from build123d import *

# Parameters (mm, degrees)
SKETCH_1_W          = 9
SKETCH_1_H          = 6.5
EXTRUDE_1_DEPTH     = 400
SKETCH_2_R          = 1.75
CUT_EXTRUDE_1_DEPTH = 7.5
SKETCH_3_R          = 3
CUT_EXTRUDE_2_DEPTH = 3.5
CUT_EXTRUDE_3_DEPTH = 401
SKETCH_5_R          = 1.75
CUT_EXTRUDE_4_DEPTH = 10


with BuildPart() as part:
    # 草图1 → 凸台-拉伸1 (new body)
    with BuildSketch(Plane.XY):
        Rectangle(SKETCH_1_W, SKETCH_1_H)
    extrude(amount=EXTRUDE_1_DEPTH)

    # 草图2 → 切除-拉伸1 (cut, through all)
    with BuildSketch(Plane(origin=(0, 3.25, 0), x_dir=(1, 0, 0), z_dir=(0, 1, 0))):
        with Locations((0, -7.5)):
            Circle(SKETCH_2_R)
        with Locations((0, -27.5)):
            Circle(SKETCH_2_R)
        with Locations((0, -47.5)):
            Circle(SKETCH_2_R)
        with Locations((0, -67.5)):
            Circle(SKETCH_2_R)
        with Locations((0, -87.5)):
            Circle(SKETCH_2_R)
        with Locations((0, -107.5)):
            Circle(SKETCH_2_R)
        with Locations((0, -127.5)):
            Circle(SKETCH_2_R)
        with Locations((0, -147.5)):
            Circle(SKETCH_2_R)
        with Locations((0, -167.5)):
            Circle(SKETCH_2_R)
        with Locations((0, -187.5)):
            Circle(SKETCH_2_R)
        with Locations((0, -207.5)):
            Circle(SKETCH_2_R)
        with Locations((0, -227.5)):
            Circle(SKETCH_2_R)
        with Locations((0, -247.5)):
            Circle(SKETCH_2_R)
        with Locations((0, -267.5)):
            Circle(SKETCH_2_R)
        with Locations((0, -287.5)):
            Circle(SKETCH_2_R)
        with Locations((0, -307.5)):
            Circle(SKETCH_2_R)
        with Locations((0, -327.5)):
            Circle(SKETCH_2_R)
        with Locations((0, -347.5)):
            Circle(SKETCH_2_R)
        with Locations((0, -367.5)):
            Circle(SKETCH_2_R)
    extrude(amount=-CUT_EXTRUDE_1_DEPTH, mode=Mode.SUBTRACT)

    # 草图3 → 切除-拉伸2 (cut)
    with BuildSketch(Plane(origin=(0, 3.25, 0), x_dir=(1, 0, 0), z_dir=(0, 1, 0))):
        with Locations((0, -7.5)):
            Circle(SKETCH_3_R)
        with Locations((0, -27.5)):
            Circle(SKETCH_3_R)
        with Locations((0, -47.5)):
            Circle(SKETCH_3_R)
        with Locations((0, -67.5)):
            Circle(SKETCH_3_R)
        with Locations((0, -87.5)):
            Circle(SKETCH_3_R)
        with Locations((0, -107.5)):
            Circle(SKETCH_3_R)
        with Locations((0, -127.5)):
            Circle(SKETCH_3_R)
        with Locations((0, -147.5)):
            Circle(SKETCH_3_R)
        with Locations((0, -167.5)):
            Circle(SKETCH_3_R)
        with Locations((0, -187.5)):
            Circle(SKETCH_3_R)
        with Locations((0, -207.5)):
            Circle(SKETCH_3_R)
        with Locations((0, -227.5)):
            Circle(SKETCH_3_R)
        with Locations((0, -247.5)):
            Circle(SKETCH_3_R)
        with Locations((0, -267.5)):
            Circle(SKETCH_3_R)
        with Locations((0, -287.5)):
            Circle(SKETCH_3_R)
        with Locations((0, -307.5)):
            Circle(SKETCH_3_R)
        with Locations((0, -327.5)):
            Circle(SKETCH_3_R)
        with Locations((0, -347.5)):
            Circle(SKETCH_3_R)
        with Locations((0, -367.5)):
            Circle(SKETCH_3_R)
        with Locations((0, -387.5)):
            Circle(SKETCH_3_R)
    extrude(amount=-CUT_EXTRUDE_2_DEPTH, mode=Mode.SUBTRACT)

    # 草图4 → 切除-拉伸3 (cut, through all)
    with BuildSketch(Plane(origin=(0, 0, 0), x_dir=(-1, 0, 0), z_dir=(0, 0, -1))):
        Polygon((4.5, -0.25), (3.5, -0.45), (3.5, -1.05), (4.5, -1.25), align=None)
        Polygon((-4.5, -0.25), (-3.5, -0.45), (-3.5, -1.05), (-4.5, -1.25), align=None)
    extrude(amount=-CUT_EXTRUDE_3_DEPTH, mode=Mode.SUBTRACT)

    # 草图5 → 切除-拉伸4 (cut)
    with BuildSketch(Plane(origin=(0, -0.25, 0), x_dir=(1, 0, 0), z_dir=(0, 1, 0))):
        with Locations((0, -387.5)):
            Circle(SKETCH_5_R)
    extrude(amount=-CUT_EXTRUDE_4_DEPTH, mode=Mode.SUBTRACT)


solid = part.part
Geometry check sheet. Reference: the model listing, model coordinates, mm. Give positions to 0.01 mm unless a question says otherwise; leave off trailing zeros. Loops run counter-clockwise (first coordinate to the right, second up) from the corner with the lowest first, then second, coordinate; pieces in that order, holes last. Notation, with made-up numbers: (73, 57.5) -> (78, 57.5) arc R18 cw to (78, 91.5) -> close; hole circle Ø1 at (-37, 40). An arc over 180 degrees is marked (long way). Answer in a Markdown table with one row per item. Add a question column.
1) Cross-section at B-B on z = 221. Record the boundary of the cut face in (x, y).
2) Gauge pin test, flat ends, axial feed: P1, Ø4.5, axis at x = 0, z = 107.5, coming from the +Y side; P2, Ø3, axis at x = 0, z = 327.5, coming from the +Y side. Record the tip position at first contact, or that the pin passes through.
3) Material ranges on probe 1 along X at (y, z) = (-1.35, 247.5); probe 2 along X at (y, z) = (0.95, 267.5); probe 3 along Y at (x, z) = (3.75, 177.5), recorded low to high. Write a range as from..to.
4) Cross-section at A-A on y = 1.75. State how many separate pieces and enclosed holes the cut face has, and give its area (3 significant figures).
Outcome:
| question | item | result |
|---|---|---|
| 1 | outline | (-4.5, -3.25) -> (4.5, -3.25) -> (4.5, -1.25) -> (3.5, -1.05) -> (3.5, -0.45) -> (4.5, -0.25) -> (4.5, 3.25) -> (-4.5, 3.25) -> (-4.5, -0.25) -> (-3.5, -0.45) -> (-3.5, -1.05) -> (-4.5, -1.25) -> close |
| 2 | P1 | stops at y = -0.25 |
| 2 | P2 | passes through |
| 3 | probe 1 | x = -4.5..-1.75, 1.75..4.5 |
| 3 | probe 2 | x = -4.5..-3, 3..4.5 |
| 3 | probe 3 | y = -3.25..-1.1, -0.4..3.25 |
| 4 | separate pieces | 1 |
| 4 | enclosed holes | 20 |
| 4 | area | 3,030 mm^2 |
